from build123d import *

# Parameters (mm, degrees)
SKETCH1_W                    = 70
SKETCH1_H                    = 40
SKETCH1_R                    = 7.6
BOSS_EXTRUDE1_DEPTH          = 80
FILLET1_R                    = 10
CUT_EXTRUDE_THIN1_DEPTH      = 1
CUT_EXTRUDE_THIN1_DEPTH_BACK = 95
SKETCH24_W                   = 28.832930408
SKETCH24_H                   = 56
CUT_EXTRUDE15_DEPTH          = 39
CUT_EXTRUDE15_DEPTH_BACK     = 40
CUT_EXTRUDE17_DEPTH          = 5
SKETCH28_R                   = 1.95
CUT_EXTRUDE18_DEPTH          = 20
MIRROR2_COPY_1_DEPTH         = 5
MIRROR2_COPY_2_SKETCH_R      = 1.95
MIRROR2_COPY_2_DEPTH         = 20


with BuildPart() as part:
    # Sketch1 → Boss-Extrude1 (new body)
    with BuildSketch(Plane.XY):
        with Locations((25, 0)):
            Rectangle(SKETCH1_W, SKETCH1_H)
        Circle(SKETCH1_R, mode=Mode.SUBTRACT)
        with Locations((50, 0)):
            Circle(SKETCH1_R, mode=Mode.SUBTRACT)
    extrude(amount=BOSS_EXTRUDE1_DEPTH)

    # Fillet1
    fillet1_edges = [part.edges().sort_by_distance(p)[0] for p in [
        (25, -20, 80),
        (25, -20, 0),
        (25, 20, 0),
        (25, 20, 80),
    ]]
    fillet(fillet1_edges, radius=FILLET1_R)

    # Sketch12 → Cut-Extrude-Thin1 (cut, two sides)
    with BuildSketch(Plane.XY.offset(80)) as cut_extrude_thin1_sk:
        Polygon((3.119310539, -0.5), (7.6, -0.5), (42.4, -0.5), (46.98201893, -0.5), (46.98201893, 0.5), (42.4, 0.5), (7.6, 0.5), (3.119310539, 0.5), align=None)
    extrude(amount=CUT_EXTRUDE_THIN1_DEPTH, mode=Mode.SUBTRACT)
    extrude(cut_extrude_thin1_sk.sketch, amount=-CUT_EXTRUDE_THIN1_DEPTH_BACK, mode=Mode.SUBTRACT)

    # Sketch24 → Cut-Extrude15 (cut, two sides)
    with BuildSketch(Plane.XZ.offset(-0.5)) as cut_extrude15_sk:
        with Locations((25, 40)):
            Rectangle(SKETCH24_W, SKETCH24_H)
    extrude(amount=CUT_EXTRUDE15_DEPTH, mode=Mode.SUBTRACT)
    extrude(cut_extrude15_sk.sketch, amount=-CUT_EXTRUDE15_DEPTH_BACK, mode=Mode.SUBTRACT)

    # Sketch27 → Cut-Extrude17 (cut)
    with BuildSketch(Plane(origin=(0, 20, 0), x_dir=(1, 0, 0), z_dir=(0, 1, 0))):
        with BuildLine():
            Line((-10, -10), (0, -10))
            ThreePointArc((0, -10), (3.535533906, -11.464466094), (5, -15))
            Line((5, -15), (5, -65))
            ThreePointArc((5, -65), (3.535533906, -68.535533906), (0, -70))
            Line((0, -70), (-10, -70))
            Line((-10, -70), (-10, -10))
        make_face()
    cut_extrude17 = extrude(amount=-CUT_EXTRUDE17_DEPTH, mode=Mode.SUBTRACT)

    # Sketch28 → Cut-Extrude18 (cut)
    with BuildSketch(Plane(origin=(0, 15, 0), x_dir=(1, 0, 0), z_dir=(0, 1, 0))):
        with Locations((-2.5, -15)):
            Circle(SKETCH28_R)
        with Locations((-2.5, -40)):
            Circle(SKETCH28_R)
        with Locations((-2.5, -65)):
            Circle(SKETCH28_R)
    cut_extrude18 = extrude(amount=-CUT_EXTRUDE18_DEPTH, mode=Mode.SUBTRACT)

    # Mirror1: Cut-Extrude17, Cut-Extrude18 across plane
    add(cut_extrude17.mirror(Plane.ZY.offset(-25)), mode=Mode.SUBTRACT)
    add(cut_extrude18.mirror(Plane.ZY.offset(-25)), mode=Mode.SUBTRACT)

    # Mirror2: Cut-Extrude17, Cut-Extrude18 across plane
    add(cut_extrude17.mirror(Plane.ZX), mode=Mode.SUBTRACT)
    add(cut_extrude18.mirror(Plane.ZX), mode=Mode.SUBTRACT)

    # Mirror2 copy 1 sketch → Mirror2 copy 1 (cut)
    with BuildSketch(Plane(origin=(50, -20, 0), x_dir=(-1, 0, 0), z_dir=(0, -1, 0))):
        with BuildLine():
            Line((-10, -10), (0, -10))
            ThreePointArc((0, -10), (3.535533906, -11.464466094), (5, -15))
            Line((5, -15), (5, -65))
            ThreePointArc((5, -65), (3.535533906, -68.535533906), (0, -70))
            Line((0, -70), (-10, -70))
            Line((-10, -70), (-10, -10))
        make_face()
    extrude(amount=-MIRROR2_COPY_1_DEPTH, mode=Mode.SUBTRACT)

    # Mirror2 copy 2 sketch → Mirror2 copy 2 (cut)
    with BuildSketch(Plane(origin=(50, -15, 0), x_dir=(-1, 0, 0), z_dir=(0, -1, 0))):
        with Locations((-2.5, -15)):
            Circle(MIRROR2_COPY_2_SKETCH_R)
        with Locations((-2.5, -40)):
            Circle(MIRROR2_COPY_2_SKETCH_R)
        with Locations((-2.5, -65)):
            Circle(MIRROR2_COPY_2_SKETCH_R)
    extrude(amount=-MIRROR2_COPY_2_DEPTH, mode=Mode.SUBTRACT)


solid = part.part
Read the model definition and answer for the solid it produces. Units are mm, in the model's axes. A direction names the side the tool comes from. Round coordinates to 2 decimals unless told otherwise and drop trailing zeros. Write each loop counter-clockwise with the first axis right and the second up, starting at its lowest first coordinate (ties: lowest second). Pieces come first, ordered by that corner, then holes. Notation, with made-up numbers: (3, 4.5) - (20, 4.5) arc R23 cw to (20, 25.5) - close; hole circle Ø3 at (17, -7.75). An arc over 180 degrees is marked (long way). One line per question, with ' | ' between items. Start each with the question number.
1. Each of these flat-tipped pins is pushed along its axis until it touches: pin 1 (4 mm diameter, centred on x = 12.5, y = -14, fed in from -Z); pin 2 (5.5 mm diameter, centred on x = 55.5, y = -16.5, fed in from +Z); pin 3 (3 mm diameter, centred on x = 52.5, z = 15, fed in from -Y) (3 decimals); pin 4 (5.5 mm diameter, centred on x = 54, y = -16.5, fed in from -Z). Where does it stop, or does it pass through?
2. For faces 4 (the face through (-5, -18, 10)), 5 (the face through (49, -15, 40)), 6 (the face through (3, 18, 11)), determine the directions among +Z, -Z, +X, -X, +Y, -Y from which every point of the face is accessible in a straight line to the end or side of a thin tool.
3. For a pull along Z with two mould halves and no side action, classify faces 1 (the face through (25.49, 17.15, 76.99)), 2 (the face through (60, 0, 39)), 3 (the face through (4, -18, 68)) as +Z half, -Z half, draft (parallel to the pull), parting line (faces both ways), or undercut.
4. Section C-C (y = -9) is taken. Determine the outline of the cut face in (x, z).
5. Section B-B (x = 21) is taken. Determine the outline of the cut face in (y, z), and give its area (3 significant figures).
6. Section A-A (z = 54) is taken. Determine the outline of the cut face in (x, y).
7. Find the intervals of material crossed by probe 1 along X at (y, z) = (-9, 40); probe 2 along Z at (x, y) = (-2.5, 10.5); probe 3 along Y at (x, z) = (49.5, 12.5), in increasing order. Write a range as [from, to].
8. Section D-D (z = 39) is taken. Give the number of separate pieces and of enclosed holes in the cut face, and give its area (3 significant figures).
Filled in:
1) pin 1: z = 0.2 | pin 2: z = 79.27 | pin 3: through | pin 4: z = 0.73
2) face 4: -X, -Y | face 5: +X, -Y | face 6: -X, +Y
3) face 1: +Z half | face 2: draft | face 3: undercut
4) outline: (-10, 0) - (60, 0) - (60, 80) - (-10, 80) - close; hole circle Ø3.9 at (-2.5, 15); hole circle Ø3.9 at (-2.5, 40); hole circle Ø3.9 at (-2.5, 65); hole (10.58, 12) - (39.42, 12) - (39.42, 68) - (10.58, 68) - close; hole circle Ø3.9 at (52.5, 15); hole circle Ø3.9 at (52.5, 40); hole circle Ø3.9 at (52.5, 65)
5) outline: (-20, 10) arc R10 ccw to (-10, 0) - (-0.5, 0) - (-0.5, 12) - (-20, 12) - close; (-20, 68) - (-0.5, 68) - (-0.5, 80) - (-10, 80) arc R10 ccw to (-20, 70) - close; (0.5, 0) - (10, 0) arc R10 ccw to (20, 10) - (20, 12) - (0.5, 12) - close; (0.5, 68) - (20, 68) - (20, 70) arc R10 ccw to (10, 80) - (0.5, 80) - close | area: 850 mm²
6) outline: (-10, -15) - (5, -15) - (5, -20) - (10.58, -20) - (10.58, -0.5) - (7.58, -0.5) arc R7.6 cw (long way) to (7.58, 0.5) - (10.58, 0.5) - (10.58, 20) - (5, 20) - (5, 15) - (-10, 15) - close; (39.42, -20) - (45, -20) - (45, -15) - (60, -15) - (60, 15) - (45, 15) - (45, 20) - (39.42, 20) - (39.42, 0.5) - (42.42, 0.5) arc R7.6 cw (long way) to (42.42, -0.5) - (39.42, -0.5) - close
7) probe 1: [-10, -4.45], [-0.55, 10.58], [39.42, 50.55], [54.45, 60] | probe 2: [0.01, 13.05], [16.95, 38.05], [41.95, 63.05], [66.95, 79.99] | probe 3: [-15, -7.58], [7.58, 15]
8) separate pieces: 6 | enclosed holes: 0 | area: 872 mm²
